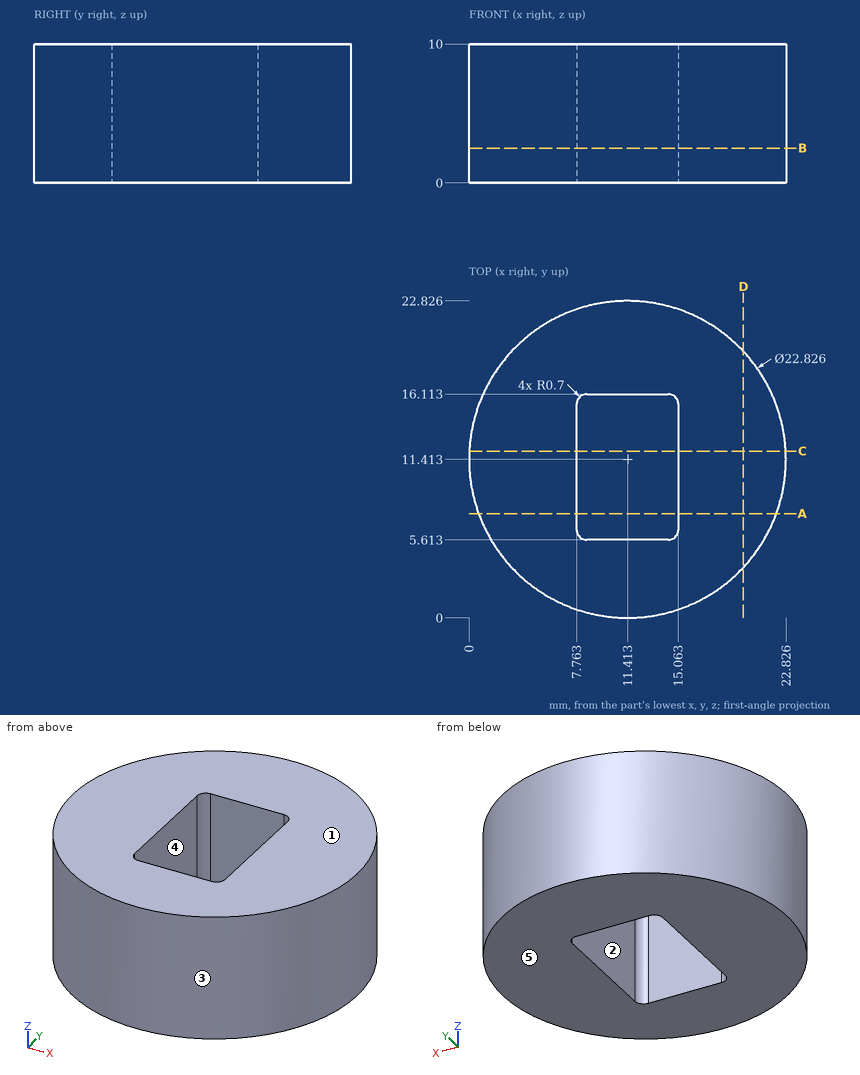
Study the drawing (mm; zero at the part's minimum x, y, z) and answer. A direction names the side the tool comes from. Round coordinates to 2 decimals unless told otherwise and drop trailing zeros. Write each loop counter-clockwise with the first axis right and the second up, starting at its lowest first coordinate (ties: lowest second). Pieces come first, ordered by that corner, then holes. Notation, with made-up numbers: (68, 2) -> (101, 2) arc R23 ccw to (101, 24) -> close; hole circle Ø6 at (18, 2). An arc over 180 degrees is marked (long way). Write item = value, one per line.
1) Section B-B on z = 2.5 is taken. Write down the section's boundary in (x, y) (1 decimal).
Check values:
outline = circle Ø22.8 at (11.4, 11.4); hole (7.8, 6.3) arc R0.7 ccw to (8.5, 5.6) -> (14.4, 5.6) arc R0.7 ccw to (15.1, 6.3) -> (15.1, 15.4) arc R0.7 ccw to (14.4, 16.1) -> (8.5, 16.1) arc R0.7 ccw to (7.8, 15.4) -> close
2) For a pull along X with two mould halves and no side action, classify the marked faces 3, 4 and 5 as released by +X, released by -X, zero draft, split by the parting line, or undercut.
Check values:
face_3 = split by the parting line
face_4 = undercut
face_5 = zero draft
3) Section C-C on y = 12 is taken. Write down the section's boundary in (x, z) (1 decimal), plus the area to 3 significant figures.
Check values:
outline = (0, 0) -> (7.8, 0) -> (7.8, 10) -> (0, 10) -> close; (15.1, 0) -> (22.8, 0) -> (22.8, 10) -> (15.1, 10) -> close
area = 155 mm²
4) Given pin 1 (1.5 mm diameter, centred on x = 7, z = 2, fed in from +Y); pin 2 (3 mm diameter, centred on y = 2.5, z = 6, fed in from -X) (1 decimal); pin 3 (1 mm diameter, centred on y = 14.5, z = 6, fed in from +X); pin 4 (1 mm diameter, centred on x = 9, y = 13.5, fed in from -Z), each flat-ended and moving along its own axis, determine where each tip first touches the part or whether it passes through.
Check values:
pin_1 = 22.22
pin_2 = 2.7
pin_3 = 22.53
pin_4 = through
5) Straight lines are drawn through the part: line 1 along X through (y, z) = (11.25, 6.25) (1 decimal); line 2 along Y through (x, z) = (10, 7.25); line 3 along Y through (x, z) = (9, 7). For each, find the intervals that lie inside material, in ascending order. Write a range as [from, to].
Check values:
line_1 = [0, 7.8], [15.1, 22.8]
line_2 = [0.09, 5.61], [16.11, 22.74]
line_3 = [0.26, 5.61], [16.11, 22.57]
6) Which of the six approach directions +Z, -Z, +X, -X, +Y, -Y give full straight-line access (tool end or side, diameter ignored) to the marked faces 1 and 2?
Check values:
face_1 = +Z, +X, -X, +Y, -Y
face_2 = +Z, -Z
7) Section D-D on x = 19.75 is taken. Write down the section's boundary in (y, z), plus the area to 3 significant figures.
Check values:
outline = (3.62, 0) -> (19.21, 0) -> (19.21, 10) -> (3.62, 10) -> close
area = 156 mm²
8) Section A-A on y = 7.5 is taken. Write down the section's boundary in (x, z).
Check values:
outline = (0.69, 0) -> (7.76, 0) -> (7.76, 10) -> (0.69, 10) -> close; (15.06, 0) -> (22.13, 0) -> (22.13, 10) -> (15.06, 10) -> close
